Could you check a few things on this model? Use its own coordinates, in mm. A direction names the side the tool comes from. Round coordinates to 2 decimals unless told otherwise and drop trailing zeros. Write each loop counter-clockwise with the first axis right and the second up, starting at its lowest first coordinate (ties: lowest second). Pieces come first, ordered by that corner, then holes. Notation, with made-up numbers: (58.25, -23.5) - (80.25, -23.5) arc R31 cw to (80.25, 6.5) - close; hole circle Ø2 at (21.25, 8.5). An arc over 180 degrees is marked (long way). Put each result on its own line as item: value.
from build123d import *

# Parameters (mm, degrees)
CROQUIS1_R              = 1
CROQUIS1_W              = 3.35
CROQUIS1_H              = 3.35
CROQUIS1_W_2            = 4.4
CROQUIS1_H_2            = 16.2
SALIENTE_EXTRUIR1_DEPTH = 2


with BuildPart() as part:
    # Croquis1 → Saliente-Extruir1 (new body)
    with BuildSketch(Plane.XY):
        with BuildLine():
            Line((-3, 3), (-3, 18.6))
            ThreePointArc((-3, 18.6), (-2.443502884, 19.943502884), (-1.1, 20.5))
            Line((-1.1, 20.5), (1.1, 20.5))
            ThreePointArc((1.1, 20.5), (2.443502884, 19.943502884), (3, 18.6))
            Line((3, 18.6), (3, 3))
            Line((3, 3), (18.6, 3))
            ThreePointArc((18.6, 3), (19.943502884, 2.443502884), (20.5, 1.1))
            Line((20.5, 1.1), (20.5, -1.1))
            ThreePointArc((20.5, -1.1), (19.943502884, -2.443502884), (18.6, -3))
            Line((18.6, -3), (3, -3))
            Line((3, -3), (3, -18.6))
            ThreePointArc((3, -18.6), (2.443502884, -19.943502884), (1.1, -20.5))
            Line((1.1, -20.5), (-1.1, -20.5))
            ThreePointArc((-1.1, -20.5), (-2.443502884, -19.943502884), (-3, -18.6))
            Line((-3, -18.6), (-3, -3))
            Line((-3, -3), (-18.6, -3))
            ThreePointArc((-18.6, -3), (-19.943502884, -2.443502884), (-20.5, -1.1))
            Line((-20.5, -1.1), (-20.5, 1.1))
            ThreePointArc((-20.5, 1.1), (-19.943502884, 2.443502884), (-18.6, 3))
            Line((-18.6, 3), (-3, 3))
        make_face()
        with Locations((0, 18.5)):
            Circle(CROQUIS1_R, mode=Mode.SUBTRACT)
        with Locations((18.5, 0)):
            Circle(CROQUIS1_R, mode=Mode.SUBTRACT)
        with Locations((0, -18.5)):
            Circle(CROQUIS1_R, mode=Mode.SUBTRACT)
        with Locations((-18.5, 0)):
            Circle(CROQUIS1_R, mode=Mode.SUBTRACT)
        with Locations((0, -13.5)):
            Rectangle(CROQUIS1_W, CROQUIS1_H, mode=Mode.SUBTRACT)
        Rectangle(CROQUIS1_W_2, CROQUIS1_H_2, mode=Mode.SUBTRACT)
    extrude(amount=SALIENTE_EXTRUIR1_DEPTH)


solid = part.part
(1) Please list where these lines run through material, in increasing order: probe 1 along Y at (x, z) = (0, 1.25) (3 decimals); probe 2 along Y at (x, z) = (-18.5, 0.6); probe 3 along Y at (x, z) = (9, 0.95). Write a range as from..to.
Values found:
probe 1: y = -20.5..-19.5, -17.5..-15.175, -11.825..-8.1, 8.1..17.5, 19.5..20.5
probe 2: y = -3..-1, 1..3
probe 3: y = -3..3
(2) Imagine slicing it at B-B, the plane z = 1.3. Give the number of separate pieces and of enclosed holes in the cut face, then the cut area to 3 significant figures.
Values found:
separate pieces: 1
enclosed holes: 6
area: 355 mm^2
(3) If we mould it in two halves opening along X, with no side actions, what happens to faces 1 (the face through (-19.958, 2.429, 0.986)), 2 (the face through (-11, 3, 1)), 3 (the face through (-0.217, 17.524, 0.986)), 4 (the face through (-0.217, -19.476, 0.986))? For each: pulls with the +X half, pulls with the -X half, needs draft (parallel to the pull), parting line crosses it, or undercut.
Values found:
face 1: pulls with the -X half
face 2: needs draft
face 3: undercut
face 4: undercut
(4) Imagine slicing it at A-A, the plane x = 0. List the corners of the cut face in (y, z) for me (3 decimals).
Values found:
outline: (-20.5, 0) - (-19.5, 0) - (-19.5, 2) - (-20.5, 2) - close; (-17.5, 0) - (-15.175, 0) - (-15.175, 2) - (-17.5, 2) - close; (-11.825, 0) - (-8.1, 0) - (-8.1, 2) - (-11.825, 2) - close; (8.1, 0) - (17.5, 0) - (17.5, 2) - (8.1, 2) - close; (19.5, 0) - (20.5, 0) - (20.5, 2) - (19.5, 2) - close
(5) For faces 5 (the face through (3, 11, 1)), 6 (the face through (0, -15.175, 1)), 7 (the face through (-3, 11, 1)), which set-ups out of +Z, -Z, +X, -X, +Y, -Y let a thin tool reach every point of the face, with its end or its side?
Values found:
face 5: +Z, -Z, +X, +Y
face 6: +Z, -Z
face 7: +Z, -Z, -X, +Y
(6) I'm going to push a flat-ended pin straight in: pin 1 (0.6 mm diameter, centred on y = -10.5, z = 0.5, fed in from +X). Where does the tip first touch, or does it pass through?
Values found:
pin 1: stops at x = 3
(7) Imagine slicing it at C-C, the plane y = 0. List the corners of the cut face in (x, z) for me, then the cut area to 3 significant figures.
Values found:
outline: (-20.5, 0) - (-19.5, 0) - (-19.5, 2) - (-20.5, 2) - close; (-17.5, 0) - (-2.2, 0) - (-2.2, 2) - (-17.5, 2) - close; (2.2, 0) - (17.5, 0) - (17.5, 2) - (2.2, 2) - close; (19.5, 0) - (20.5, 0) - (20.5, 2) - (19.5, 2) - close
area: 65.2 mm^2
(8) Imagine slicing it at D-D, the plane y = -12.5. List the corners of the cut face in (x, z) for me (3 decimals).
Values found:
outline: (-3, 0) - (-1.675, 0) - (-1.675, 2) - (-3, 2) - close; (1.675, 0) - (3, 0) - (3, 2) - (1.675, 2) - close
